Work out the finished part from the listing and answer in its coordinate system (mm). Face numbers are marked on the shaded views. A direction names the side the tool comes from. Give positions to 0.01 mm unless a question says otherwise; leave off trailing zeros. Order: outer loops, then holes, each group sorted by start corner. A loop starts at its lowest first (then second) coordinate and runs counter-clockwise, first axis right, second up. Notation, with made-up numbers: M 79.5,-28.5 L 92.5,-28.5 A17 ccw 92.5,-12.5 Z; hole C 11.5,82 d5. An arc over 180 degrees is marked long. One line per item, written item: value.
from build123d import *

# Parameters (mm, degrees)
BASE_FLANGE1_DEPTH             = 2.65684
EDGE_FLANGE2_STRIP_W           = 16.97736
EDGE_FLANGE2_STRIP_H           = 2.65684
EDGE_FLANGE2_STRIP_CUT_DEPTH   = 85.842119192
EDGE_FLANGE2_STRIP_2_W         = 16.97736
EDGE_FLANGE2_STRIP_2_H         = 2.65684
EDGE_FLANGE2_STRIP_CUT_2_DEPTH = 85.842119192
EDGE_FLANGE2_DEPTH             = 85.842119192
EDGE_FLANGE2_BEND_DEPTH        = 85.842119192
SKETCH22_W                     = 2.65684
SKETCH22_H                     = 35
BOSS_EXTRUDE1_DEPTH            = 36.846685
SKETCH24_W                     = 2.65684
SKETCH24_H                     = 35
BOSS_EXTRUDE2_DEPTH            = 36.846685
EDGE_FLANGE3_STRIP_CUT_DEPTH   = 35
EDGE_FLANGE3_DEPTH             = 35
EDGE_FLANGE4_STRIP_CUT_DEPTH   = 35
EDGE_FLANGE4_DEPTH             = 35
SKETCH32_R                     = 2.75
CUT_EXTRUDE1_DEPTH             = 198.310511697
FILLET1_R                      = 3


# Sheet-metal steps are written as plain solids
with BuildPart() as part:
    # Sketch4 → Base-Flange1 (new body)
    with BuildSketch(Plane(origin=(0, 95.2, 0), x_dir=(1, 0, 0), z_dir=(0, 1, 0))):
        Polygon((-55.697100796, -148.712214058), (-46.070125043, -151.418011142), (46.070125043, -151.418011142), (55.697100796, -148.712214058), (32.469965214, -66.072214058), (22.842989462, -68.778011142), (-22.842989462, -68.778011142), (-32.469965214, -66.072214058), align=None)
        with BuildLine():
            Line((-26.32, -128.668011142), (-26.32, -138.668011142))
            ThreePointArc((-26.32, -138.668011142), (-23.57, -141.418011142), (-20.82, -138.668011142))
            Line((-20.82, -138.668011142), (-20.82, -128.668011142))
            ThreePointArc((-20.82, -128.668011142), (-23.57, -125.918011142), (-26.32, -128.668011142))
        make_face(mode=Mode.SUBTRACT)
        with BuildLine():
            Line((20.82, -128.668011142), (20.82, -138.668011142))
            ThreePointArc((20.82, -138.668011142), (23.57, -141.418011142), (26.32, -138.668011142))
            Line((26.32, -138.668011142), (26.32, -128.668011142))
            ThreePointArc((26.32, -128.668011142), (23.57, -125.918011142), (20.82, -128.668011142))
        make_face(mode=Mode.SUBTRACT)
        with BuildLine():
            Line((20.82, -91.528011142), (20.82, -81.528011142))
            ThreePointArc((20.82, -81.528011142), (23.57, -78.778011142), (26.32, -81.528011142))
            Line((26.32, -81.528011142), (26.32, -91.528011142))
            ThreePointArc((26.32, -91.528011142), (23.57, -94.278011142), (20.82, -91.528011142))
        make_face(mode=Mode.SUBTRACT)
        with BuildLine():
            Line((-19.25, -105.098011142), (-19.25, -115.098011142))
            ThreePointArc((-19.25, -115.098011142), (0, -134.348011142), (19.25, -115.098011142))
            Line((19.25, -115.098011142), (19.25, -105.098011142))
            ThreePointArc((19.25, -105.098011142), (0, -85.848011142), (-19.25, -105.098011142))
        make_face(mode=Mode.SUBTRACT)
        with BuildLine():
            Line((-20.82, -91.528011142), (-20.82, -81.528011142))
            ThreePointArc((-20.82, -81.528011142), (-23.57, -78.778011142), (-26.32, -81.528011142))
            Line((-26.32, -81.528011142), (-26.32, -91.528011142))
            ThreePointArc((-26.32, -91.528011142), (-23.57, -94.278011142), (-20.82, -91.528011142))
        make_face(mode=Mode.SUBTRACT)
    extrude(amount=-BASE_FLANGE1_DEPTH)

    # Edge-Flange2 strip (across the edge) → Edge-Flange2 strip cut (cut)
    with BuildSketch(Plane(origin=(32.469965214, 92.54316, 66.072214058), x_dir=(-0.9626975752484609, -3.4914813388431334e-15, 0.2705797084238469), z_dir=(0.2705797084238469, 0, 0.9626975752484609))):
        with Locations((-5.31368, -1.32842)):
            Rectangle(EDGE_FLANGE2_STRIP_W, EDGE_FLANGE2_STRIP_H)
    extrude(amount=EDGE_FLANGE2_STRIP_CUT_DEPTH, mode=Mode.SUBTRACT)

    # Edge-Flange2 strip 2 (across the edge) → Edge-Flange2 strip cut 2 (cut)
    with BuildSketch(Plane(origin=(-55.697100796, 92.54316, 148.712214058), x_dir=(0.9626975752484602, -3.4914813388431334e-15, 0.2705797084238493), z_dir=(0.2705797084238493, 0, -0.9626975752484602))):
        with Locations((-5.31368, -1.32842)):
            Rectangle(EDGE_FLANGE2_STRIP_2_W, EDGE_FLANGE2_STRIP_2_H)
    extrude(amount=EDGE_FLANGE2_STRIP_CUT_2_DEPTH, mode=Mode.SUBTRACT)

    # Edge-Flange2 section (across the edge) → Edge-Flange2 (add)
    with BuildSketch(Plane(origin=(32.469965214, 92.54316, 66.072214058), x_dir=(-0.9626975752484609, -3.4914813388431334e-15, 0.2705797084238469), z_dir=(0.2705797084238469, 0, 0.9626975752484609))):
        with BuildLine():
            Line((-2.65684, 3.175), (-2.65684, 42.84316))
            Line((-2.65684, 42.84316), (0, 42.84316))
            Line((0, 42.84316), (0, 3.175))
            ThreePointArc((0, 3.175), (0.92993597, 0.92993597), (3.175, 0))
            Line((3.175, 0), (3.175, -2.65684))
            ThreePointArc((3.175, -2.65684), (-0.948733611, -0.948733611), (-2.65684, 3.175))
        make_face()
    extrude(amount=EDGE_FLANGE2_DEPTH)

    # Edge-Flange2 section 2 (across the edge) → Edge-Flange2 bend (add)
    with BuildSketch(Plane(origin=(-55.697100796, 92.54316, 148.712214058), x_dir=(0.9626975752484602, -3.4914813388431334e-15, 0.2705797084238493), z_dir=(0.2705797084238493, 0, -0.9626975752484602))):
        with BuildLine():
            Line((-2.65684, 3.175), (-2.65684, 42.84316))
            Line((-2.65684, 42.84316), (0, 42.84316))
            Line((0, 42.84316), (0, 3.175))
            ThreePointArc((0, 3.175), (0.92993597, 0.92993597), (3.175, 0))
            Line((3.175, 0), (3.175, -2.65684))
            ThreePointArc((3.175, -2.65684), (-0.948733611, -0.948733611), (-2.65684, 3.175))
        make_face()
    extrude(amount=EDGE_FLANGE2_BEND_DEPTH)

    # Sketch22 → Boss-Extrude1 (add)
    with BuildSketch(Plane(origin=(19.588150967, 0, 69.69282933), x_dir=(-0.9626975752484609, 0, 0.2705797084238468), z_dir=(-0.2705797084238468, 0, -0.9626975752484609))):
        with Locations((-14.709376365, 67.2)):
            Rectangle(SKETCH22_W, SKETCH22_H)
    extrude(amount=BOSS_EXTRUDE1_DEPTH)

    # Sketch24 → Boss-Extrude2 (add)
    with BuildSketch(Plane(origin=(-19.588150967, 0, 69.69282933), x_dir=(-0.9626975752484602, 0, -0.27057970842384926), z_dir=(0.27057970842384926, 0, -0.9626975752484602))):
        with Locations((14.709376365, 67.2)):
            Rectangle(SKETCH24_W, SKETCH24_H)
    extrude(amount=BOSS_EXTRUDE2_DEPTH)

    # Edge-Flange3 strip (across the edge) → Edge-Flange3 strip cut (cut)
    with BuildSketch(Plane(origin=(25.057733426, 49.7, 29.881113007), x_dir=(1, 0, 0), z_dir=(0, 1, 0))):
        Polygon((-7.033027346, 15.203794832), (-2.439298227, -1.140268474), (0.118435199, -0.421381482), (-4.47529392, 15.922681824), align=None)
    extrude(amount=EDGE_FLANGE3_STRIP_CUT_DEPTH, mode=Mode.SUBTRACT)

    # Edge-Flange3 section (across the edge) → Edge-Flange3 (add)
    with BuildSketch(Plane(origin=(25.057733426, 49.7, 29.881113007), x_dir=(1, 0, 0), z_dir=(0, 1, 0))):
        with BuildLine():
            Line((-2.65684, 0.437709092), (-2.65684, 19.281113007))
            Line((-2.65684, 19.281113007), (0, 19.281113007))
            Line((0, 19.281113007), (0, 0.437709092))
            ThreePointArc((0, 0.437709092), (0.029748162, 0.004101115), (0.118435199, -0.421381482))
            Line((0.118435199, -0.421381482), (-2.439298227, -1.140268474))
            ThreePointArc((-2.439298227, -1.140268474), (-2.602198575, -0.35874204), (-2.65684, 0.437709092))
        make_face()
    extrude(amount=EDGE_FLANGE3_DEPTH)

    # Edge-Flange4 strip (across the edge) → Edge-Flange4 strip cut (cut)
    with BuildSketch(Plane(origin=(-25.057733426, 84.7, 29.881113007), x_dir=(-1, 0, 0), z_dir=(0, -1, 0))):
        Polygon((-7.033027346, 15.203794832), (-2.439298227, -1.140268474), (0.118435199, -0.421381482), (-4.47529392, 15.922681824), align=None)
    extrude(amount=EDGE_FLANGE4_STRIP_CUT_DEPTH, mode=Mode.SUBTRACT)

    # Edge-Flange4 section (across the edge) → Edge-Flange4 (add)
    with BuildSketch(Plane(origin=(-25.057733426, 84.7, 29.881113007), x_dir=(-1, 0, 0), z_dir=(0, -1, 0))):
        with BuildLine():
            Line((-2.65684, 0.437709092), (-2.65684, 19.281113007))
            Line((-2.65684, 19.281113007), (0, 19.281113007))
            Line((0, 19.281113007), (0, 0.437709092))
            ThreePointArc((0, 0.437709092), (0.029748162, 0.004101115), (0.118435199, -0.421381482))
            Line((0.118435199, -0.421381482), (-2.439298227, -1.140268474))
            ThreePointArc((-2.439298227, -1.140268474), (-2.602198575, -0.35874204), (-2.65684, 0.437709092))
        make_face()
    extrude(amount=EDGE_FLANGE4_DEPTH)

    # Sketch32 → Cut-Extrude1 (cut, through all)
    with BuildSketch(Plane(origin=(25.057733426, 0, 0), x_dir=(0, 0, -1), z_dir=(1, 0, 0))):
        with Locations(Location((-18.35, 77.45, 0), (0, 0, 180))):
            Circle(SKETCH32_R)
        with Locations(Location((-18.35, 57.45, 0), (0, 0, 180))):
            Circle(SKETCH32_R)
    extrude(amount=-CUT_EXTRUDE1_DEPTH, mode=Mode.SUBTRACT)

    # Fillet1
    fillet1_edges = [part.edges().sort_by_distance(p)[0] for p in [
        (56.975967508, 49.7, 148.352770562),
        (-22.842989462, 93.87158, 68.778011142),
        (22.842989462, 93.87158, 68.778011142),
        (46.070125043, 93.87158, 151.418011142),
        (-46.070125043, 93.87158, 151.418011142),
        (-56.975967508, 49.7, 148.352770562),
        (33.748831927, 84.7, 65.712770562),
        (-33.748831927, 84.7, 65.712770562),
        (23.729313426, 49.7, 10.6),
        (23.729313426, 84.7, 10.6),
        (-23.729313426, 84.7, 10.6),
        (-23.729313426, 49.7, 10.6),
    ]]
    fillet(fillet1_edges, radius=FILLET1_R)


solid = part.part
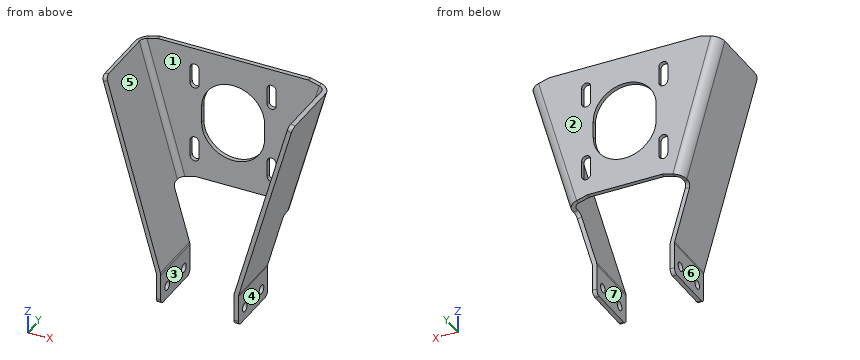
(1) Section D-D, the plane z = 36.5 is taken. Give the vertices of the cut face in (x, y), then the cut area to 3 significant figures.
Findings:
outline: M -26.92,49.7 L -24.16,49.7 L -24.16,84.7 L -26.92,84.7 Z; M 24.16,49.7 L 26.92,49.7 L 26.92,84.7 L 24.16,84.7 Z
area: 193 mm^2
(2) Given P1, Ø9.5, axis at y = 65, z = 22.5, coming from the +X side; P2, Ø4.5, axis at y = 57.45, z = 18.35, coming from the -X side; P3, Ø15, axis at y = 58.5, z = 18, coming from the -X side; P4, Ø0.8, axis at y = 94, z = 111, coming from the -X side, each flat-ended and moving along its own axis, determine where each tip first touches the part or whether it passes through.
Findings:
P1: stops at x = 25.06
P2: passes through
P3: stops at x = -25.06
P4: stops at x = -45.98
(3) Section A-A, the plane y = 77.45 is taken. Give the number of separate pieces and of enclosed holes in the cut face, then the cut area to 3 significant figures.
Findings:
separate pieces: 4
enclosed holes: 0
area: 727 mm^2
(4) Section C-C, the plane x = 0 is taken. Give the vertices of the cut face in (y, z).
Findings:
outline: M 92.54,68.78 L 95.2,68.78 L 95.2,85.85 L 92.54,85.85 Z; M 92.54,134.35 L 95.2,134.35 L 95.2,151.42 L 92.54,151.42 Z
(5) Which of the six approach directions +Z, -Z, +X, -X, +Y, -Y give full straight-line access (tool end or side, diameter ignored) to the marked faces 1, 2 and 3?
Findings:
face 1: +Z, -Y
face 2: +Z, -Z, +X, -X, +Y
face 3: +Z, -Z, +Y, -Y
(6) Find the intervals of material crossed by probe 1 along Y at (x, z) = (-23, 18); probe 2 along Y at (x, z) = (-3, 83.5); probe 3 along X at (y, z) = (56, 91.5), in increasing order. Write a range as from..to.
Findings:
probe 1: y = 49.7..54.72, 60.18..74.72, 80.18..84.7
probe 2: y = 92.54..95.2
probe 3: x = -42.38..-39.62, 39.62..42.38
(7) Section B-B, the plane z = 18.35 is taken. Give the vertices of the cut face in (x, y), then the cut area to 3 significant figures.
Findings:
outline: M -25.06,49.7 L -22.4,49.7 L -22.4,54.7 L -25.06,54.7 Z; M -25.06,60.2 L -22.4,60.2 L -22.4,74.7 L -25.06,74.7 Z; M -25.06,80.2 L -22.4,80.2 L -22.4,84.7 L -25.06,84.7 Z; M 22.4,49.7 L 25.06,49.7 L 25.06,54.7 L 22.4,54.7 Z; M 22.4,60.2 L 25.06,60.2 L 25.06,74.7 L 22.4,74.7 Z; M 22.4,80.2 L 25.06,80.2 L 25.06,84.7 L 22.4,84.7 Z
area: 128 mm^2
(8) Determine the mould class of the marked faces 4, 5, 6 and 7 for opening direction X: pulls with the +X half, pulls with the -X half, needs draft (parallel to the pull), parting line crosses it, or undercut.
Findings:
face 4: pulls with the +X half
face 5: undercut
face 6: pulls with the -X half
face 7: undercut
